```python
from build123d import *

# Parameters (mm, degrees)
CROQUIS1_R              = 1.75
CROQUIS1_R_2            = 1.05
CROQUIS1_R_3            = 1.65
CROQUIS1_R_4            = 7
CROQUIS1_W              = 22.4
CROQUIS1_H              = 12
CROQUIS1_W_2            = 3.8
CROQUIS1_H_2            = 2.3
CROQUIS1_W_3            = 6
CROQUIS1_H_3            = 20
CROQUIS1_W_4            = 45
CROQUIS1_H_4            = 45
SALIENTE_EXTRUIR1_DEPTH = 2


with BuildPart() as part:
    # Croquis1 → Saliente-Extruir1 (new body)
    with BuildSketch(Plane(origin=(0, 0, 0), x_dir=(1, 0, 0), z_dir=(0, 1, 0))):
        with BuildLine():
            Line((-50, -30), (65, -30))
            ThreePointArc((65, -30), (68.535533906, -28.535533906), (70, -25))
            ThreePointArc((70, -25), (64.574669497, -20.968704233), (61.402899266, -15))
            Line((61.402899266, -15), (61.402899266, 15))
            ThreePointArc((61.402899266, 15), (64.574669497, 20.968704233), (70, 25))
            ThreePointArc((70, 25), (68.535533906, 28.535533906), (65, 30))
            Line((65, 30), (-50, 30))
            ThreePointArc((-50, 30), (-64.142135624, 24.142135624), (-70, 10))
            Line((-70, 10), (-70, -10))
            ThreePointArc((-70, -10), (-64.142135624, -24.142135624), (-50, -30))
        make_face()
        with Locations(Location((-59, -14, 0), (0, 0, 270))):
            Circle(CROQUIS1_R, mode=Mode.SUBTRACT)
        with Locations(Location((-59, 14, 0), (0, 0, 90))):
            Circle(CROQUIS1_R, mode=Mode.SUBTRACT)
        with Locations(Location((55.730399266, 0, 0), (0, 0, 270))):
            Circle(CROQUIS1_R_2, mode=Mode.SUBTRACT)
        with Locations(Location((27.730399266, 0, 0), (0, 0, 270))):
            Circle(CROQUIS1_R_2, mode=Mode.SUBTRACT)
        with Locations(Location((-44, 0, 0), (0, 0, 270))):
            Circle(CROQUIS1_R_3, mode=Mode.SUBTRACT)
        with Locations(Location((11.88, 0, 0), (0, 0, 270))):
            Circle(CROQUIS1_R_3, mode=Mode.SUBTRACT)
        with Locations(Location((-59, 0, 0), (0, 0, 270))):
            Circle(CROQUIS1_R_4, mode=Mode.SUBTRACT)
        with Locations(Location((23.702899266, 0, 0), (0, 0, 270))):
            Circle(CROQUIS1_R_3, mode=Mode.SUBTRACT)
        with Locations((41.730399266, 0)):
            Rectangle(CROQUIS1_W, CROQUIS1_H, mode=Mode.SUBTRACT)
        with Locations((30, 26.35)):
            Rectangle(CROQUIS1_W_2, CROQUIS1_H_2, mode=Mode.SUBTRACT)
        with Locations((58, 26.35)):
            Rectangle(CROQUIS1_W_2, CROQUIS1_H_2, mode=Mode.SUBTRACT)
        with Locations((58, -26.35)):
            Rectangle(CROQUIS1_W_2, CROQUIS1_H_2, mode=Mode.SUBTRACT)
        with Locations((30, -26.35)):
            Rectangle(CROQUIS1_W_2, CROQUIS1_H_2, mode=Mode.SUBTRACT)
        with Locations((17.402899266, 0)):
            Rectangle(CROQUIS1_W_3, CROQUIS1_H_3, mode=Mode.SUBTRACT)
        with Locations((-16.095990361, 0)):
            Rectangle(CROQUIS1_W_4, CROQUIS1_H_4, mode=Mode.SUBTRACT)
    extrude(amount=SALIENTE_EXTRUIR1_DEPTH)


solid = part.part
```
Geometry: final body of the model. Coordinates: model frame, mm. A direction names the side the tool comes from. Round coordinates to 2 decimals unless told otherwise and drop trailing zeros. Write each loop counter-clockwise with the first axis right and the second up, starting at its lowest first coordinate (ties: lowest second). Pieces come first, ordered by that corner, then holes. Notation, with made-up numbers: (45.5, -38) -> (52.5, -38) arc R17 ccw to (52.5, -32) -> close; hole circle Ø3 at (-32, 25.5). An arc over 180 degrees is marked (long way). Return JSON: item names as keys, results as strings.
Q1. Set-up query: faces 1 (the cylindrical face through (-57.29, 0.99, -13.62)), 2 (the cylindrical face through (64.513, 0.986, -20.896)). Return all of +Z, -Z, +X, -X, +Y, -Y with unobstructed straight access to the full face (end or side cutting, diameter ignored); none if empty.
From the geometry:
{"face 1": "+Y, -Y", "face 2": "+X, +Y, -Y"}
Q2. Section A-A on x = 11.88. Return the cut outline in (y, z), and give its area (3 significant figures).
From the geometry:
{"outline": "(0, -30) -> (2, -30) -> (2, -1.65) -> (0, -1.65) -> close; (0, 1.65) -> (2, 1.65) -> (2, 30) -> (0, 30) -> close", "area": "113 mm2"}
Q3. Section B-B on z = 13.5. Return the cut outline in (x, y), and give its area (3 significant figures).
From the geometry:
{"outline": "(-69.69, 0) -> (-60.68, 0) -> (-60.68, 2) -> (-69.69, 2) -> close; (-57.32, 0) -> (-38.6, 0) -> (-38.6, 2) -> (-57.32, 2) -> close; (6.4, 0) -> (61.4, 0) -> (61.4, 2) -> (6.4, 2) -> close", "area": "165 mm2"}
Q4. First-contact query: pin 1 Ø0.6 at (y, z) = (1, -4) entering from +X; pin 2 Ø1.7 at (x, z) = (27.73, 0) entering from -Y. Flat tips, straight axial feed; report the tip coordinate or a pass-through.
From the geometry:
{"pin 1": "x = 61.4", "pin 2": "through"}
Q5. Mould query, pull axis X, two halves, no side actions, for faces 3 (the cylindrical face through (-64.297, 0.986, 23.986)), 4 (the flat face through (15, 0, -14)), 5 (the cylindrical face through (10.27, 0.99, -0.36)). Classes: +X half, -X half, draft (parallel to the pull), parting line (faces both ways), or undercut.
From the geometry:
{"face 3": "-X half", "face 4": "draft", "face 5": "undercut"}
Q6. Ray query, line 1 (Z direction, x = 58.5, y = 1.25); line 2 (Z direction, x = -23, y = 0.6); line 3 (X direction, y = 0.8, z = 7.5). Return the intervals inside material, ascending.
From the geometry:
{"line 1": "-30 to -27.5, -25.2 to 25.2, 27.5 to 30", "line 2": "-30 to -22.5, 22.5 to 30", "line 3": "-70 to -38.6, 6.4 to 14.4, 20.4 to 61.4"}
Q7. Section D-D on x = -36. Return the cut outline in (y, z), and give its area (3 significant figures).
From the geometry:
{"outline": "(0, -30) -> (2, -30) -> (2, -22.5) -> (0, -22.5) -> close; (0, 22.5) -> (2, 22.5) -> (2, 30) -> (0, 30) -> close", "area": "30.0 mm2"}
Q8. Section C-C on x = -59. Return the cut outline in (y, z), and give its area (3 significant figures).
From the geometry:
{"outline": "(0, -27.86) -> (2, -27.86) -> (2, -15.75) -> (0, -15.75) -> close; (0, -12.25) -> (2, -12.25) -> (2, -7) -> (0, -7) -> close; (0, 7) -> (2, 7) -> (2, 12.25) -> (0, 12.25) -> close; (0, 15.75) -> (2, 15.75) -> (2, 27.86) -> (0, 27.86) -> close", "area": "69.4 mm2"}
